from build123d import *

# Parameters (mm, degrees)
MODEL_W             = 5.5
MODEL_H             = 5.5
BOSS_EXTRUDE1_DEPTH = 6


with BuildPart() as part:
    # Model → Boss-Extrude1 (new body)
    with BuildSketch(Plane.XY):
        with BuildLine():
            Line((3055.225160199, 1463.457958964), (3055.225160199, 1448.457958964))
            Line((3055.225160199, 1448.457958964), (3067.725160199, 1448.457958964))
            Line((3067.725160199, 1448.457958964), (3067.725160199, 1442.457958964))
            Line((3067.725160199, 1442.457958964), (3073.725160199, 1442.457958964))
            Line((3073.725160199, 1442.457958964), (3073.725160199, 1448.457958964))
            Line((3073.725160199, 1448.457958964), (3076.225160199, 1448.457958964))
            Line((3076.225160199, 1448.457958964), (3076.225160199, 1479.457958964))
            Line((3076.225160199, 1479.457958964), (3068.475988022, 1479.457958964))
            ThreePointArc((3068.475988022, 1479.457958964), (3106.225160199, 1504.457958964), (3143.974332375, 1479.457958964))
            Line((3143.974332375, 1479.457958964), (3136.225160199, 1479.457958964))
            Line((3136.225160199, 1479.457958964), (3136.225160199, 1448.457958964))
            Line((3136.225160199, 1448.457958964), (3147.225160199, 1448.457958964))
            Line((3147.225160199, 1448.457958964), (3157.225160199, 1448.457958964))
            Line((3157.225160199, 1448.457958964), (3157.225160199, 1463.457958964))
            ThreePointArc((3157.225160199, 1463.457958964), (3106.225160199, 1514.457958964), (3055.225160199, 1463.457958964))
        make_face()
        with Locations((3141.725160199, 1453.957958964)):
            Rectangle(MODEL_W, MODEL_H, mode=Mode.SUBTRACT)
        with Locations((3141.725160199, 1473.957958964)):
            Rectangle(MODEL_W, MODEL_H, mode=Mode.SUBTRACT)
        with Locations((3070.725160199, 1453.957958964)):
            Rectangle(MODEL_W, MODEL_H, mode=Mode.SUBTRACT)
        with Locations((3070.725160199, 1473.957958964)):
            Rectangle(MODEL_W, MODEL_H, mode=Mode.SUBTRACT)
    extrude(amount=BOSS_EXTRUDE1_DEPTH)


solid = part.part
For this review, take the finished solid that the model builds, in its own axes (mm). A direction names the side the tool comes from. Round coordinates to 2 decimals unless told otherwise and drop trailing zeros. Write each loop counter-clockwise with the first axis right and the second up, starting at its lowest first coordinate (ties: lowest second). Pieces come first, ordered by that corner, then holes. Notation, with made-up numbers: (8, -16.5) - (15, -16.5) arc R18 ccw to (15, 9.5) - close; hole circle Ø1 at (-28, -20.75). An arc over 180 degrees is marked (long way). Write item = value, one per line. Start each with the question number.
1. Consider section A-A on y = 1497. State the section outline as (x, z) points.
2. For faces 4 (the face through (3073.475, 1454, 3)), 5 (the face through (3076.225, 1464, 3)), 6 (the face through (3067.725, 1445, 3)), 7 (the face through (3102, 1505, 6)), 8 (the face through (3075, 1448.458, 3)), list the 3-axis set-ups (+Z, -Z, +X, -X, +Y, -Y) from which the entire face can be reached by the end or side of a thin tool; tool diameter is ignored.
3. Draft analysis for pull direction Y (two halves, no side actions). For faces 1 (the face through (3136.225, 1464, 3)), 2 (the face through (3071, 1442.458, 3)), 3 (the face through (3073.475, 1474, 3)), state which applies: released by +Y, released by -Y, zero draft, split by the parting line, or undercut.
4. Consider section D-D on x = 3071. State the section outline as (y, z) points, plus the area to 3 significant figures.
5. Wall thickness on L1, parallel to X at y = 1446, z = 1.9; L2, parallel to X at y = 1498, z = 4; L3, parallel to X at y = 1490, z = 1.4: over which ranges is each line inside the solid? List them lowest first.
6. Consider section B-B on z = 2.5. Give the number of separate pieces and of enclosed holes in the cut face, plus the area to 3 significant figures.
7. For pin 1 Ø1.5 at (x, z) = (3126, 4.5) entering from +Y; pin 2 Ø3 at (x, z) = (3140.5, 4) entering from +Y; pin 3 Ø3 at (x, z) = (3071.5, 2) entering from +Y, all flat-tipped, find the tip position at first contact; note any pin that passes through.
8. Consider section C-C on x = 3137.5. State the section outline as (y, z) points.
Evaluation:
q1.outline = (3067.81, 0) - (3082.65, 0) - (3082.65, 6) - (3067.81, 6) - close; (3129.8, 0) - (3144.64, 0) - (3144.64, 6) - (3129.8, 6) - close
q2.face_4 = +Z, -Z
q2.face_5 = +Z, -Z, -Y
q2.face_6 = +Z, -Z, -X, -Y
q2.face_7 = +Z, +X, -X, +Y, -Y
q2.face_8 = +Z, -Z, +X, -Y
q3.face_1 = zero draft
q3.face_2 = released by -Y
q3.face_3 = undercut
q4.outline = (1442.46, 0) - (1451.21, 0) - (1451.21, 6) - (1442.46, 6) - close; (1456.71, 0) - (1471.21, 0) - (1471.21, 6) - (1456.71, 6) - close; (1476.71, 0) - (1479.46, 0) - (1479.46, 6) - (1476.71, 6) - close; (1484.44, 0) - (1500.34, 0) - (1500.34, 6) - (1484.44, 6) - close
q4.area = 251 mm2
q5.L1 = 3067.73 to 3073.73
q5.L2 = 3068.7 to 3084.14, 3128.31 to 3143.75
q5.L3 = 3062.68 to 3074.98, 3137.47 to 3149.77
q6.separate_pieces = 1
q6.enclosed_holes = 4
q6.area = 2,310 mm2
q7.pin_1 = 1510.78
q7.pin_2 = 1502.53
q7.pin_3 = 1502.15
q8.outline = (1448.46, 0) - (1479.46, 0) - (1479.46, 6) - (1448.46, 6) - close; (1489.97, 0) - (1503.74, 0) - (1503.74, 6) - (1489.97, 6) - close
